Could you check a few things on this drawing? It's one solid part, dimensions in mm from its lowest x, y, z. Give positions to 0.01 mm unless a question says otherwise; leave off trailing zeros. Loops run counter-clockwise (first coordinate to the right, second up) from the corner with the lowest first, then second, coordinate; pieces in that order, holes last. Notation, with made-up numbers: (39, -1.5) - (79, -1.5) arc R25 ccw to (79, 35.5) - close; hole circle Ø1 at (87.5, -20.5). An arc over 180 degrees is marked (long way). Write each question's results on one line, items separated by ' | '. Start each with the question number.
(1) I need wall thicknesses on line 1 (Z direction, x = 81, y = 72.5); line 2 (Y direction, x = 47, z = 6); line 3 (Y direction, x = 43, z = 6.75) (1 decimal). Which ranges of each line are inside material? Lowest first, please.
(2) If we mould it in two halves opening along X, with no side actions, what happens to the marked faces 1, 2 and 3? For each: released by +X, released by -X, zero draft, split by the parting line, or undercut.
(3) Suppose I cut it at C-C (y = 28.5). Please give me the cut outline in (x, z).
(4) For pin 1 (2 mm diameter, centred on y = 73.5, z = 4.5, fed in from -X); pin 2 (2 mm diameter, centred on y = 32, z = 2, fed in from +X); pin 3 (5 mm diameter, centred on x = 39, y = 84.5, fed in from +Z), each with a flat end and sliding along its axis, tell me the tip position at first contact or that it passes through.
(5) Suppose I cut it at A-A (y = 53). Please give me the cut outline in (x, z).
(6) Suppose I cut it at B-B (x = 32). Please give me the cut outline in (y, z), and give its area (3 significant figures).
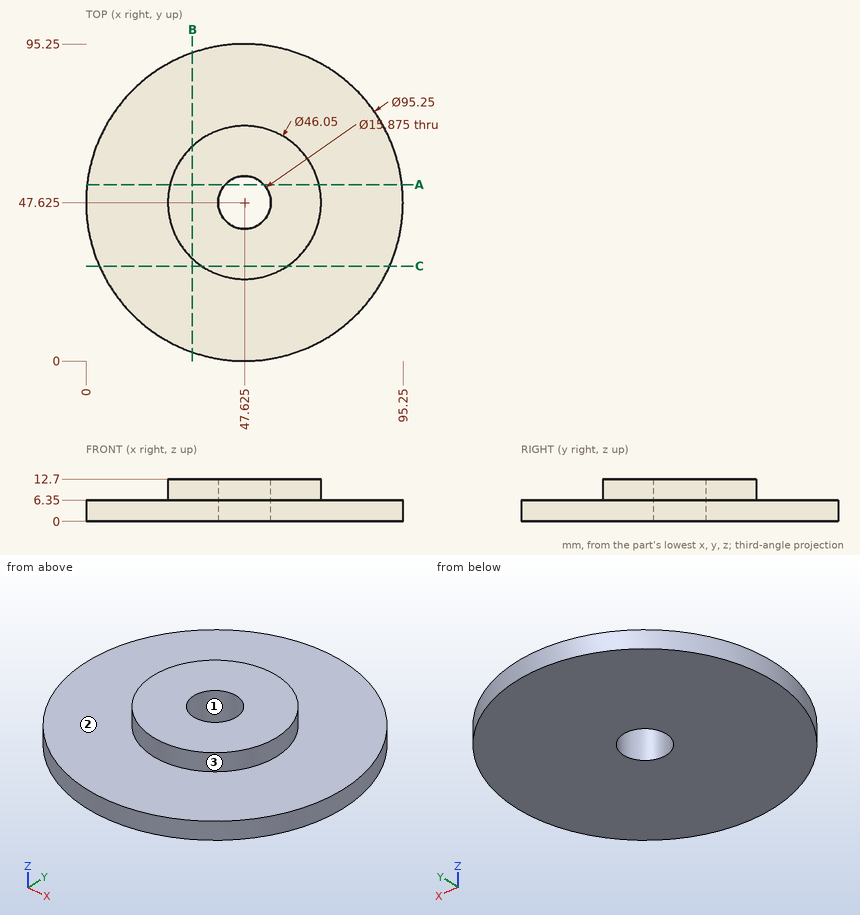
Output values:
1) line 1: 0 to 6.35 | line 2: 0 to 39.71, 55.54 to 95.25 | line 3: 25.1 to 41.2, 54.1 to 70.2
2) face 1: undercut | face 2: zero draft | face 3: split by the parting line
3) outline: (4.01, 0) - (91.24, 0) - (91.24, 6.35) - (60.45, 6.35) - (60.45, 12.7) - (34.8, 12.7) - (34.8, 6.35) - (4.01, 6.35) - close
4) pin 1: x = 7.01 | pin 2: x = 92.95 | pin 3: z = 6.35
5) outline: (0.3, 0) - (41.78, 0) - (41.78, 12.7) - (25.24, 12.7) - (25.24, 6.35) - (0.3, 6.35) - close; (53.47, 0) - (94.95, 0) - (94.95, 6.35) - (70.01, 6.35) - (70.01, 12.7) - (53.47, 12.7) - close
6) outline: (2.64, 0) - (92.61, 0) - (92.61, 6.35) - (64.54, 6.35) - (64.54, 12.7) - (30.71, 12.7) - (30.71, 6.35) - (2.64, 6.35) - close | area: 786 mm2
